from build123d import *

# Parameters (mm, degrees)
F0_R     = 101.6
F1_DEPTH = 9.525
F3_DEPTH = 9.526
F4_R     = 6.35


with BuildPart() as f1:
    # F0 (on Top) → F1 (new body)
    with BuildSketch(Plane.XY):
        Circle(F0_R)
    extrude(amount=F1_DEPTH)

    # F2 (on face) → F3 (cut, through all)
    with BuildSketch(Plane.XY.offset(9.525)):
        with BuildLine():
            Line((6.35, -101.401368334), (6.35, -24.5934442484))
            ThreePointArc((6.35, -24.5934442484), (0, 25.4), (-6.35, -24.5934442484))
            Line((-6.35, -24.5934442484), (-6.35, -101.401368334))
            ThreePointArc((-6.35, -101.401368334), (0, -101.6), (6.35, -101.401368334))
        make_face()
    extrude(amount=-F3_DEPTH, mode=Mode.SUBTRACT)

    # F4
    f4_edges = [f1.edges().sort_by_distance(p)[0] for p in [
        (-6.35, -101.401368, 4.7625),
        (6.35, -101.401368, 4.7625),
        (-6.35, -24.593444, 4.7625),
        (6.35, -24.593444, 4.7625),
    ]]
    fillet(f4_edges, radius=F4_R)


solid = f1.part
Work out the finished part from the listing and answer in its coordinate system (mm). A direction names the side the tool comes from. Round coordinates to 2 decimals unless told otherwise and drop trailing zeros. Order: outer loops, then holes, each group sorted by start corner. A loop starts at its lowest first (then second) coordinate and runs counter-clockwise, first axis right, second up. Notation, with made-up numbers: M 88,-37.75 L 119,-37.75 A26 cw 119,-17.75 Z; hole C 27.25,22 d6. An arc over 180 degrees is marked long. Put each result on its own line as item: value. Start each with the question number.
Q1. For a pull along X with two mould halves and no side action, classify faces 4 (the flat face through (6.35, -62, 5)), 5 (the cylindrical face through (4.28, 101.51, 4.7)), 6 (the cylindrical face through (0.97, 25.38, 4.83)), 7 (the flat face through (21, -21, 9.525)) as pulls with the +X half, pulls with the -X half, needs draft (parallel to the pull), parting line crosses it, or undercut.
Q2. Section B-B, the plane z = 6.25 is taken. Write down the section's boundary in (x, y), and give its area (3 significant figures).
Q3. Straight lines are drawn through the part: L1, parallel to X at y = 0, z = 7; L2, parallel to Y at x = 0, z = 4.75; L3, parallel to X at y = -50.5, z = 3.5. For each, find the intervals that lie inside material, in ascending order. Write a range as [from, to].
Q4. Section D-D, the plane x = 0 is taken. Write down the section's boundary in (y, z) (3 decimals).
Q5. A flat-ended cylindrical pin translates along its axis: pin 1 (3 mm diameter, centred on y = -47.5, z = 4.5, fed in from +X). Find the tip coordinate at first contact, or state that the pin passes through.
Q6. Section A-A, the plane y = 0 is taken. Write down the section's boundary in (x, z) (3 decimals).
Q7. Section C-C, the plane y = -43.5 is taken. Write down the section's boundary in (x, z) (3 decimals).
Q8. A tool of negligible diameter and unlimited length cuts with its end or side. For faces 1 (the flat face through (21, -21, 0)), 2 (the cylindrical face through (-7.36, -25.66, 4.7)), 3 (the flat face through (-6.35, -61, 5)), from which of +Z, -Z, +X, -X, +Y, -Y can it reach the whole face along a straight path? Write none if from no direction.
Findings below:
1. face 4: undercut
1. face 5: parting line crosses it
1. face 6: undercut
1. face 7: needs draft
2. outline: M -13.55,-100.69 A6.35 ccw -6.35,-94.4 L -6.35,-29.1 A6.35 ccw -10.16,-23.28 A25.4 cw long 10.16,-23.28 A6.35 ccw 6.35,-29.1 L 6.35,-94.4 A6.35 ccw 13.55,-100.69 A101.6 ccw long Z
2. area: 29,400 mm^2
3. L1: x = [-101.6, -25.4], [25.4, 101.6]
3. L2: y = [25.4, 101.6]
3. L3: x = [-88.16, -6.35], [6.35, 88.16]
4. outline: M 25.4,0 L 101.6,0 L 101.6,9.525 L 25.4,9.525 Z
5. pin 1: stops at x = 90.59
6. outline: M -101.6,0 L -25.4,0 L -25.4,9.525 L -101.6,9.525 Z; M 25.4,0 L 101.6,0 L 101.6,9.525 L 25.4,9.525 Z
7. outline: M -91.817,0 L -6.35,0 L -6.35,9.525 L -91.817,9.525 Z; M 6.35,0 L 91.817,0 L 91.817,9.525 L 6.35,9.525 Z
8. face 1: -Z, +X, -X, +Y, -Y
8. face 2: +Z, -Z
8. face 3: +Z, -Z, -Y
